For this review, use the dimensioned drawing (mm, ordinates from the lowest corner) and the shaded views. A direction names the side the tool comes from. Round coordinates to 2 decimals unless told otherwise and drop trailing zeros. Write each loop counter-clockwise with the first axis right and the second up, starting at its lowest first coordinate (ties: lowest second). Pieces come first, ordered by that corner, then holes. Notation, with made-up numbers: (76.25, -5.5) - (130.25, -5.5) arc R25 cw to (130.25, 23.5) - close; hole circle Ø6 at (28, -32.75). An arc over 180 degrees is marked (long way). Write each question's results on one line, items separated by ' | '.
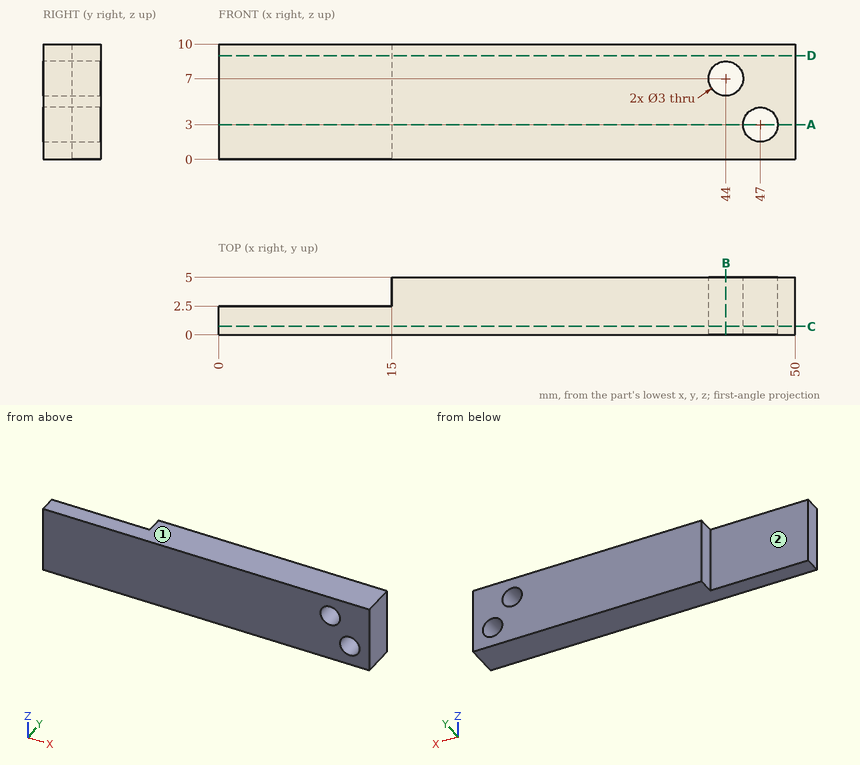
Q1. We need section D-D (z = 9). State the section outline as (x, y) points.
Evaluation:
outline: (0, 0) - (50, 0) - (50, 5) - (15, 5) - (15, 2.5) - (0, 2.5) - close
Q2. Tool access review of the marked faces 1 and 2: name each direction out of +Z, -Z, +X, -X, +Y, -Y from which nothing blocks a thin tool from reaching the whole face with its end or side.
Evaluation:
face 1: +Z, +X, -X, +Y, -Y | face 2: +Z, -Z, -X, +Y
Q3. We need section B-B (x = 44). State the section outline as (y, z) points.
Evaluation:
outline: (0, 0) - (5, 0) - (5, 5.5) - (0, 5.5) - close; (0, 8.5) - (5, 8.5) - (5, 10) - (0, 10) - close
Q4. For probe 1 along X at (y, z) = (1.1, 7); probe 2 along X at (y, z) = (2.4, 3); probe 3 along Y at (x, z) = (12, 1.5), list the stretches that pass through material, from the lowest coordinate up.
Evaluation:
probe 1: x = 0 to 42.5, 45.5 to 50 | probe 2: x = 0 to 45.5, 48.5 to 50 | probe 3: y = 0 to 2.5
Q5. We need section A-A (z = 3). State the section outline as (x, y) points, plus the area to 4 significant figures.
Evaluation:
outline: (0, 0) - (45.5, 0) - (45.5, 5) - (15, 5) - (15, 2.5) - (0, 2.5) - close; (48.5, 0) - (50, 0) - (50, 5) - (48.5, 5) - close | area: 197.5 mm^2
Q6. Insertion check: P1, Ø3, axis at x = 9.5, z = 7.5, coming from the +Y side; P2, Ø0.8, axis at y = 4, z = 3, coming from the -X side. Each pin has a flat end and moves straight along its axis. Give the tip position at first contact, or say it passes through.
Evaluation:
P1: stops at y = 2.5 | P2: stops at x = 15
Q7. We need section C-C (y = 0.75). State the section outline as (x, z) points, plus the area to 3 significant figures.
Evaluation:
outline: (0, 0) - (50, 0) - (50, 10) - (0, 10) - close; hole circle Ø3 at (44, 7); hole circle Ø3 at (47, 3) | area: 486 mm^2
